Solid Edge part; units mm, degrees
sketch "Sketch1" plane through (0, 0, 0) normal (0, -1, 0) x (1, 0, 0)
  line L0 (-55, 70) -> (55, 70)
  arc A0 (55, 70) -> (35, 50) centre (55, 50) ccw
  line L1 (35, 0) -> (35, 50)
  line L2 (-35, 0) -> (-35, 50)
  arc A1 (-55, 70) -> (-35, 50) centre (-55, 50) cw
  arc A2 (35, 0) -> (-35, 0) centre (0, 0) cw
extrude "Protrusion1" add sketch "Sketch1" against normal blind 25
sketch "Sketch2" plane through (0, 0, 17.5) normal (0, -1, 0) x (1, 0, 0)
  line L0 (-60, 132.5) -> (-35, 132.5)
  line L1 (-35, 132.5) -> (-35, 77.5)
  line L2 (-35, 77.5) -> (35, 77.5)
  line L3 (35, 77.5) -> (35, 132.5)
  line L4 (35, 132.5) -> (60, 132.5)
  line L5 (60, 132.5) -> (60, 52.5)
  line L6 (-60, 52.5) -> (60, 52.5)
  line L7 (-60, 52.5) -> (-60, 132.5)
extrude "ExtrudedProtrusion_2" add sketch "Sketch2" against normal blind 80
sketch "Sketch3" plane through (0, 0, 57.5) normal (0, -1, 0) x (1, 0, 0)
  circle A0 centre (0, -57.5) radius 15
extrude "ExtrudedCutout_1" cut sketch "Sketch3" against normal blind 25
sketch "Sketch4" plane through (60, 40, 110) normal (1, 0, 0) x (0, 0, -1)
  circle A0 centre (-12.5035, 0) radius 20
extrude "ExtrudedCutout_5" cut sketch "Sketch4" against normal blind 120
Design review of the part built by this model. Coordinates are the model's own, in mm. A direction names the side the tool comes from. Coordinates: 2 decimals unless noted, no trailing zeros. Loops run counter-clockwise (first coordinate to the right, second up) from the corner with the lowest first, then second, coordinate; pieces in that order, holes last.
Q1. For pin 1 (20 mm diameter, centred on y = 17, z = 28.5, fed in from +X); pin 2 (12 mm diameter, centred on x = -17.5, y = 29, fed in from +Z); pin 3 (7.5 mm diameter, centred on y = 13.5, z = 35.5, fed in from -X); pin 4 (1.5 mm diameter, centred on x = -33, z = -11, fed in from -Y), all flat-tipped, find the tip position at first contact; note any pin that passes through.
Reported:
pin 1: stops at x = 35
pin 2: stops at z = 95
pin 3: stops at x = -35
pin 4: stops at y = 0
Q2. We need section A-A on y = 40. State the section outline as (x, z) points.
Reported:
outline: (-60, 70) - (60, 70) - (60, 102.5) - (35, 102.5) - (35, 95) - (-35, 95) - (-35, 102.5) - (-60, 102.5) - close; (-60, 142.5) - (-35, 142.5) - (-35, 150) - (-60, 150) - close; (35, 142.5) - (60, 142.5) - (60, 150) - (35, 150) - close
Q3. Tool access review of faces 1 (the face through (1, 25, 28)), 2 (the face through (35, 31, 104)), 3 (the face through (-35, 12, 25)), 4 (the face through (35, 12, 25)): name each direction out of +Z, -Z, +X, -X, +Y, -Y from which nothing blocks a thin tool from reaching the whole face with its end or side.
Reported:
face 1: -Z, +X, -X, +Y
face 2: +Z, +Y, -Y
face 3: -Z, -X, +Y, -Y
face 4: -Z, +X, +Y, -Y
Q4. The part is to be moulded in two halves that separate along Z. For faces 5 (the face through (-1, 48, 70)), 6 (the face through (47, 39, 150)), 7 (the face through (47.68, 53.52, 137.24)), say which applies: +Z half, -Z half, draft (parallel to the pull), parting line (faces both ways), or undercut.
Reported:
face 5: -Z half
face 6: +Z half
face 7: undercut
Q5. We need section D-D on y = 63. State the section outline as (x, z) points.
Reported:
outline: (-60, 70) - (60, 70) - (60, 150) - (35, 150) - (35, 95) - (-35, 95) - (-35, 150) - (-60, 150) - close
Q6. We need section B-B on z = 98. State the section outline as (x, y) points, and give its area (3 significant figures).
Reported:
outline: (-60, 0) - (-35, 0) - (-35, 80) - (-60, 80) - close; (35, 0) - (60, 0) - (60, 80) - (35, 80) - close
area: 4,000 mm2
Q7. To check wall thickness, follow line 1 (Z direction, x = 0, y = 6); line 2 (Y direction, x = 46, z = 123); line 3 (X direction, y = 18.5, z = 100.5). State the ranges of each line that lie inside material, in increasing order.
Reported:
line 1: z = -35 to -15, 15 to 95
line 2: y = 0 to 20.01, 59.99 to 80
line 3: x = -60 to -35, 35 to 60
Q8. We need section C-C on x = 0. State the section outline as (y, z) points, and give its area (4 significant figures).
Reported:
outline: (0, -35) - (25, -35) - (25, -15) - (0, -15) - close; (0, 15) - (25, 15) - (25, 70) - (80, 70) - (80, 95) - (0, 95) - close
area: 3,875 mm2
